from build123d import *

# Parameters (mm, degrees)
BASE_EXTRUDE_DEPTH   = 30
CUT_EXTRUDE1_DEPTH   = 6
FILLET1_R            = 6
FILLET1_OF_MIRROR1_R = 6
MIRROR2_START        = -8
MIRROR2_DEPTH        = 6
MIRROR2_START_2      = 2
MIRROR2_2_DEPTH      = 6
SKETCH5_W            = 16
SKETCH5_H            = 75
CUT_EXTRUDE3_DEPTH   = 1.5
SKETCH6_W            = 10
SKETCH6_H            = 69
CUT_EXTRUDE4_DEPTH   = 18.5
CUT_EXTRUDE5_DEPTH   = 120.750782878


# Read off the part's stored shape, not the designer's step: Mirror2
with BuildPart() as part:
    # Sketch1 → Base-Extrude (new body)
    with BuildSketch(Plane(origin=(0, 0, 0), x_dir=(1, 0, 0), z_dir=(0, 1, 0))):
        with BuildLine():
            Line((8, 37.5), (2.993373056, 112.699293126))
            ThreePointArc((2.993373056, 112.699293126), (0, 115.5), (-2.993373056, 112.699293126))
            Line((-2.993373056, 112.699293126), (-8, 37.5))
            Line((-8, 37.5), (-8, -37.5))
            Line((-8, -37.5), (-2.993373056, -112.699293126))
            ThreePointArc((-2.993373056, -112.699293126), (0, -115.5), (2.993373056, -112.699293126))
            Line((2.993373056, -112.699293126), (8, -37.5))
            Line((8, -37.5), (8, 37.5))
        make_face()
    extrude(amount=BASE_EXTRUDE_DEPTH)

    # Sketch2 → Cut-Extrude1 (cut)
    with BuildSketch(Plane(origin=(8, 0, 0), x_dir=(0, 0, -1), z_dir=(1, 0, 0))):
        with BuildLine():
            Line((-37.5, 5), (-95.5, 5))
            ThreePointArc((-95.5, 5), (-105.5, 15), (-95.5, 25))
            Line((-95.5, 25), (-37.5, 25))
            Line((-37.5, 25), (-37.5, 5))
        make_face()
    cut_extrude1 = extrude(amount=-CUT_EXTRUDE1_DEPTH, mode=Mode.SUBTRACT)

    # Fillet1
    fillet1_edges = [part.edges().sort_by_distance(p)[0] for p in [
        (5, 25, 37.5),
        (5, 5, 37.5),
    ]]
    fillet(fillet1_edges, radius=FILLET1_R)

    # Mirror1: Cut-Extrude1 across plane
    add(cut_extrude1.mirror(Plane(origin=(0, 0, 0), x_dir=(0, 0, 1), z_dir=(1, 0, 0))), mode=Mode.SUBTRACT)

    # Fillet1 of Mirror1
    fillet1_of_mirror1_edges = [part.edges().sort_by_distance(p)[0] for p in [
        (-5, 25, 37.5),
        (-5, 5, 37.5),
    ]]
    fillet(fillet1_of_mirror1_edges, radius=FILLET1_OF_MIRROR1_R)

    # Mirror2 outline → Mirror2 (cut)
    with BuildSketch(Plane.YZ.offset(MIRROR2_START)):
        with BuildLine():
            Line((5, -43.5), (5, -95.5))
            ThreePointArc((5, -95.5), (15, -105.5), (25, -95.5))
            Line((25, -95.5), (25, -43.5))
            ThreePointArc((25, -43.5), (23.242640687, -39.257359313), (19, -37.5))
            Line((19, -37.5), (11, -37.5))
            ThreePointArc((11, -37.5), (6.757359313, -39.257359313), (5, -43.5))
        make_face()
    extrude(amount=MIRROR2_DEPTH, mode=Mode.SUBTRACT)

    # Mirror2 2 outline → Mirror2 2 (cut)
    with BuildSketch(Plane.YZ.offset(MIRROR2_START_2)):
        with BuildLine():
            Line((5, -43.5), (5, -95.5))
            ThreePointArc((5, -95.5), (15, -105.5), (25, -95.5))
            Line((25, -95.5), (25, -43.5))
            ThreePointArc((25, -43.5), (23.242640687, -39.257359313), (19, -37.5))
            Line((19, -37.5), (11, -37.5))
            ThreePointArc((11, -37.5), (6.757359313, -39.257359313), (5, -43.5))
        make_face()
    extrude(amount=MIRROR2_2_DEPTH, mode=Mode.SUBTRACT)

    # Sketch5 → Cut-Extrude3 (cut)
    with BuildSketch(Plane(origin=(0, 30, 0), x_dir=(-1, 0, 0), z_dir=(0, 1, 0))):
        Rectangle(SKETCH5_W, SKETCH5_H)
    extrude(amount=-CUT_EXTRUDE3_DEPTH, mode=Mode.SUBTRACT)

    # Sketch6 → Cut-Extrude4 (cut)
    with BuildSketch(Plane(origin=(0, 28.5, 0), x_dir=(1, 0, 0), z_dir=(0, 1, 0))):
        Rectangle(SKETCH6_W, SKETCH6_H)
    extrude(amount=-CUT_EXTRUDE4_DEPTH, mode=Mode.SUBTRACT)

    # Sketch7 → Cut-Extrude5 (cut, through all)
    with BuildSketch(Plane(origin=(2, 0, 0), x_dir=(0, 0, -1), z_dir=(1, 0, 0))):
        with BuildLine():
            Line((39.5, 11), (39.5, 19))
            ThreePointArc((39.5, 19), (40.671572875, 21.828427125), (43.5, 23))
            Line((43.5, 23), (95.5, 23))
            ThreePointArc((95.5, 23), (103.5, 15), (95.5, 7))
            Line((95.5, 7), (43.5, 7))
            ThreePointArc((43.5, 7), (40.671572875, 8.171572875), (39.5, 11))
        make_face()
        with BuildLine():
            Line((-95.5, 7), (-43.5, 7))
            ThreePointArc((-43.5, 7), (-40.671572875, 8.171572875), (-39.5, 11))
            Line((-39.5, 11), (-39.5, 19))
            ThreePointArc((-39.5, 19), (-40.671572875, 21.828427125), (-43.5, 23))
            Line((-43.5, 23), (-95.5, 23))
            ThreePointArc((-95.5, 23), (-103.5, 15), (-95.5, 7))
        make_face()
    extrude(amount=-CUT_EXTRUDE5_DEPTH, mode=Mode.SUBTRACT)


solid = part.part
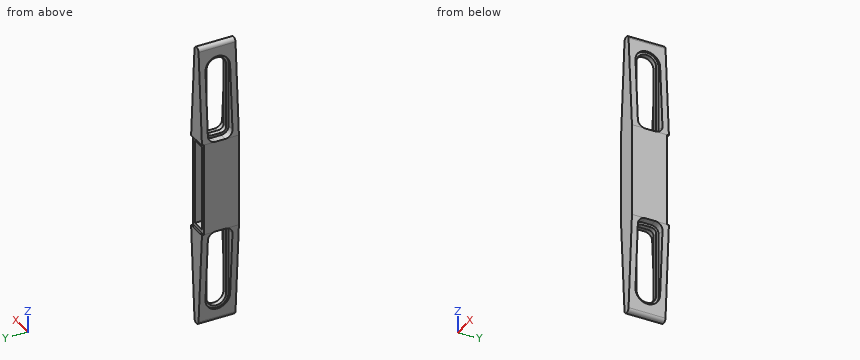
The listing builds one solid part. Answer for the finished solid, in the listing's coordinates (mm). Round coordinates to 2 decimals unless told otherwise and drop trailing zeros. Order: outer loops, then holes, each group sorted by start corner. A loop starts at its lowest first (then second) coordinate and runs counter-clockwise, first axis right, second up. Notation, with made-up numbers: M -19,-10 L 31,-10 A25 cw 31,18 Z; hole C -27,-38.75 d11. An arc over 180 degrees is marked long. Answer in a Markdown table with one row per item. Add a question column.
1) The part is cut by section A-A on x = 0. Determine the outline of the cut face in (y, z).
2) The part is cut by section D-D on z = -31.5. Determine the outline of the cut face in (x, y).
3) Flat-ended cylindrical pins translate along their axes: pin 1 Ø1.5 at (x, y) = (-2.5, 8) entering from +Z; pin 2 Ø4 at (x, y) = (3, 16.5) entering from -Z; pin 3 Ø1.2 at (x, y) = (1, 29) entering from +Z; pin 4 Ø8 at (y, z) = (16, 68.5) entering from +X. Find the tip coordinate at first contact, or state that the pin passes through.
4) The part is cut by section C-C on z = 76. Determine the outline of the cut face in (x, y), plus the area to 3 significant figures.
5) Consider line 1 along Y through (x, z) = (-4.25, -84); line 2 along Z through (x, y) = (0.5, 17.25); line 3 along Z through (x, y) = (-4, 15.5). Determine where each line is inside the solid, lowest interval first. Write a range as from..to.
6) The part is cut by section B-B on y = 15. Count the separate pieces of the cut face and the enclosed holes in it, plus the area to 3 significant figures.
Findings below:
| question | item | result |
|---|---|---|
| 1 | outline | M 0,-115.5 L 30,-115.5 L 30,-37.5 L 28.5,-37.5 L 28.5,-34.5 L 10,-34.5 L 10,34.5 L 28.5,34.5 L 28.5,37.5 L 30,37.5 L 30,115.5 L 0,115.5 Z; hole M 7,-95.5 A8 ccw 23,-95.5 L 23,-43.5 A4 ccw 19,-39.5 L 11,-39.5 A4 ccw 7,-43.5 Z; hole M 7,43.5 A4 ccw 11,39.5 L 19,39.5 A4 ccw 23,43.5 L 23,95.5 A8 ccw 7,95.5 Z |
| 2 | outline | M -8,0 L 8,0 L 8,28.5 L 5,28.5 L 5,10 L -5,10 L -5,28.5 L -8,28.5 Z |
| 3 | pin 1 | stops at z = 114.94 |
| 3 | pin 2 | stops at z = -115.33 |
| 3 | pin 3 | stops at z = 115.47 |
| 3 | pin 4 | passes through |
| 4 | outline | M -5.44,0 L 5.44,0 L 5.44,5 L 2,5 L 2,7 L -2,7 L -2,5 L -5.44,5 Z; M -5.44,25 L -2,25 L -2,23 L 2,23 L 2,25 L 5.44,25 L 5.44,30 L -5.44,30 Z |
| 4 | area | 125 mm² |
| 5 | line 1 | y = 0..5, 25..30 |
| 5 | line 2 | z = -115.46..-103.18, -39.5..-34.5, 34.5..39.5, 103.18..115.46 |
| 5 | line 3 | z = -37.5..-34.5, 34.5..37.5 |
| 6 | separate pieces | 3 |
| 6 | enclosed holes | 1 |
| 6 | area | 661 mm² |
